Could you check a few things on this model? Use its own coordinates, in mm. Round coordinates to 2 decimals unless told otherwise and drop trailing zeros. Loops run counter-clockwise (first coordinate to the right, second up) from the corner with the lowest first, then second, coordinate; pieces in that order, holes last. Notation, with made-up numbers: (-6, -28) - (50, -28) arc R20 cw to (50, 3) - close; hole circle Ø8 at (56, -22). An arc over 180 degrees is marked (long way). Put each result on its own line as item: value. Start each with the question number.
from build123d import *

# Parameters (mm, degrees)
SKETCH_1_W      = 50
SKETCH_1_H      = 20
SKETCH_1_R      = 2
EXTRUDE_1_DEPTH = 3
SKETCH_2_R      = 2
EXTRUDE_2_DEPTH = 3
FILLET_1_R      = 15


with BuildPart() as part:
    # 草图1 → 凸台-拉伸1 (new body)
    with BuildSketch(Plane.XY):
        Rectangle(SKETCH_1_W, SKETCH_1_H)
        with Locations((20, 0)):
            Circle(SKETCH_1_R, mode=Mode.SUBTRACT)
        with Locations((-20, 0)):
            Circle(SKETCH_1_R, mode=Mode.SUBTRACT)
    extrude(amount=EXTRUDE_1_DEPTH)

    # 草图2 → 凸台-拉伸2 (add)
    with BuildSketch(Plane(origin=(0, 0, 0), x_dir=(-1, 0, 0), z_dir=(0, 0, -1))):
        Polygon((-3.494170761, 10), (-14.78082372, 48.374620063), (4.406486311, 54.017946543), (17.352941176, 10), align=None)
        with Locations((-3.826468347, 46.569902088)):
            Circle(SKETCH_2_R, mode=Mode.SUBTRACT)
        with Locations((1.816858133, 27.382592056)):
            Circle(SKETCH_2_R, mode=Mode.SUBTRACT)
    extrude(amount=-EXTRUDE_2_DEPTH)

    # 圆角1
    # the kernel refuses this fillet: 15 mm, written as the material it adds along each edge
    with BuildSketch(Plane(origin=(-17.352941176, 10, 0), x_dir=(-1, 0, 0), z_dir=(0, 0, 1))) as fillet_1_piece_1:
        with BuildLine():
            CenterArc((11.360931708, -14.532967632), FILLET_1_R, 104.335036725, 59.275422941)
            Line((-3.029550815, -10.300472772), (-3.317360466, -10.215822875))
            Line((-3.317360466, -10.215822875), (-0.28780965, 0.084649897))
            Line((-0.28780965, 0.084649897), (0, 0.3))
            ThreePointArc((0, 0.3), (3.823529412, 0.3), (7.572781366, 0.290659353))
            Line((7.572781366, 0.290659353), (7.647058824, 0))
        make_face()
    extrude(amount=3)
    with BuildSketch(Plane(origin=(3.494170761, 10, 0), x_dir=(1, 0, 0), z_dir=(0, 0, 1))) as fillet_1_piece_2:
        with BuildLine():
            CenterArc((FILLET_1_R * 1.33647324392, FILLET_1_R), FILLET_1_R, 163.610459666, 106.389540334)
            Line((FILLET_1_R * 0.37710774235, FILLET_1_R * 1.28216632399), (FILLET_1_R * 0.357920432319, FILLET_1_R * 1.28780965047))
            Line((FILLET_1_R * 0.357920432319, FILLET_1_R * 1.28780965047), (-FILLET_1_R * 0.0267294648784, -FILLET_1_R * 0.02))
            Line((-FILLET_1_R * 0.0267294648784, -FILLET_1_R * 0.02), (FILLET_1_R * 1.33647324392, -FILLET_1_R * 0.02))
            Line((FILLET_1_R * 1.33647324392, -FILLET_1_R * 0.02), (FILLET_1_R * 1.33647324392, 0))
        make_face()
    extrude(amount=3)


solid = part.part
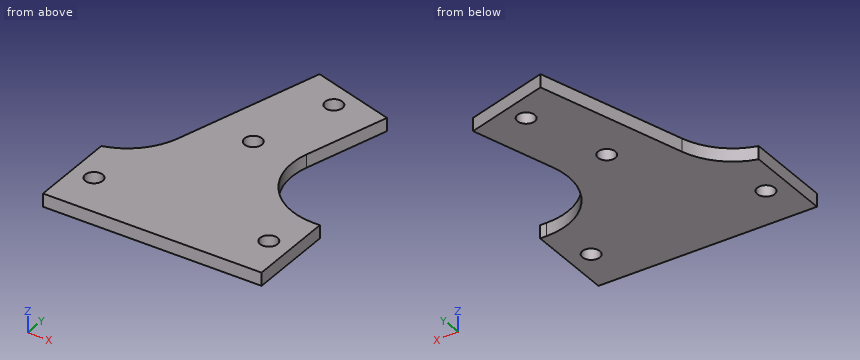
Item 1: Suppose I cut it at C-C, the plane z = 0.75. List the corners of the cut face in (x, y) for me.
Item 2: Suppose I cut it at A-A, the plane x = -3. List the corners of the cut face in (y, z) for me.
Item 3: Suppose I cut it at B-B, the plane y = 0. List the corners of the cut face in (x, z) for me, then the cut area to 3 significant figures.
Item 4: Will these pins go through, and if not, where does the flat tip stop? P1, Ø1, axis at x = 3, z = 1, coming from the +Y side; P2, Ø5, axis at x = -7, y = 47, coming from the -Z side.
Item 5: Suppose I cut it at D-D, the plane x = -20. List the corners of the cut face in (y, z) for me, then the cut area to 3 significant figures.
Item 6: I need wall thicknesses on line 1 (Y direction, x = 20, z = 0.95); line 2 (X direction, y = 46, z = 2); line 3 (X direction, y = 45.5, z = 0.9). Which ranges of each line are inside material? Lowest first, please. Write a range as from..to.
Numbers:
1. outline: (-25, -10) - (25, -10) - (25, 10) - (23.54, 10) arc R15 cw to (9.15, 29.23) - (14.78, 48.37) - (-4.41, 54.02) - (-14.32, 20.3) arc R15 cw to (-25, 10) - close; hole circle Ø4 at (-20, 0); hole circle Ø4 at (-1.82, 27.38); hole circle Ø4 at (3.83, 46.57); hole circle Ø4 at (20, 0)
2. outline: (-10, 0) - (25.77, 0) - (25.77, 3) - (-10, 3) - close; (29, 0) - (53.6, 0) - (53.6, 3) - (29, 3) - close
3. outline: (-25, 0) - (-22, 0) - (-22, 3) - (-25, 3) - close; (-18, 0) - (18, 0) - (18, 3) - (-18, 3) - close; (22, 0) - (25, 0) - (25, 3) - (22, 3) - close
3. area: 126 mm^2
4. P1: y = 51.99
4. P2: z = 0
5. outline: (-10, 0) - (-2, 0) - (-2, 3) - (-10, 3) - close; (2, 0) - (12.32, 0) - (12.32, 3) - (2, 3) - close
5. area: 55.0 mm^2
6. line 1: -10..-2, 2..10.42
6. line 2: -6.76..1.91, 5.74..14.08
6. line 3: -6.91..2.14, 5.52..13.94
